```python
from build123d import *

# Parameters (mm, degrees)
SKETCH_1_R      = 24
SKETCH_1_R_2    = 3
SKETCH_1_R_3    = 2
SKETCH_1_R_4    = 1.45
SKETCH_1_R_5    = 1.5
SKETCH_1_W      = 15.1
SKETCH_1_H      = 3
SKETCH_1_W_2    = 3
SKETCH_1_H_2    = 20.1
EXTRUDE_1_DEPTH = 2
FILLET_1_R      = 10
FILLET_2_R      = 3


with BuildPart() as part:
    # 草图1 → 凸台-拉伸1 (new body)
    with BuildSketch(Plane(origin=(0, 0, 0), x_dir=(1, 0, 0), z_dir=(0, 1, 0))):
        with BuildLine():
            Line((0, -40), (-53.115531196, -40))
            Line((-53.115531196, -40), (-53.115531196, 50))
            Line((-53.115531196, 50), (23.035101229, 50))
            ThreePointArc((23.035101229, 50), (47.273662895, 61.517967257), (61.152805225, 38.549709823))
            add(Edge.make_bspline(
                [(61.152805225, 38.549709823), (43.767754296, -41.044262003), (0, -40)],
                knots=[0, 0, 0, 0.762442078, 0.762442078, 0.762442078], degree=2))
        make_face()
        with Locations(Location((0, 0, 0), (0, 0, 270))):
            Circle(SKETCH_1_R, mode=Mode.SUBTRACT)
        with Locations(Location((41.5198, 42.363514464, 0), (0, 0, 270))):
            Circle(SKETCH_1_R_2, mode=Mode.SUBTRACT)
        with Locations(Location((46, 9, 0), (0, 0, 270))):
            Circle(SKETCH_1_R_3, mode=Mode.SUBTRACT)
        with Locations(Location((-45, 40, 0), (0, 0, 270))):
            Circle(SKETCH_1_R_3, mode=Mode.SUBTRACT)
        with Locations(Location((-45, -35, 0), (0, 0, 270))):
            Circle(SKETCH_1_R_3, mode=Mode.SUBTRACT)
        with Locations(Location((35.862945751, 48.020368713, 0), (0, 0, 270))):
            Circle(SKETCH_1_R_4, mode=Mode.SUBTRACT)
        with Locations(Location((47.176654249, 48.020368713, 0), (0, 0, 270))):
            Circle(SKETCH_1_R_4, mode=Mode.SUBTRACT)
        with Locations(Location((47.176654249, 36.706660215, 0), (0, 0, 270))):
            Circle(SKETCH_1_R_4, mode=Mode.SUBTRACT)
        with Locations(Location((35.862945751, 36.706660215, 0), (0, 0, 270))):
            Circle(SKETCH_1_R_4, mode=Mode.SUBTRACT)
        with Locations(Location((-45, 22, 0), (0, 0, 270))):
            Circle(SKETCH_1_R_5, mode=Mode.SUBTRACT)
        with Locations(Location((-45, -22, 0), (0, 0, 270))):
            Circle(SKETCH_1_R_5, mode=Mode.SUBTRACT)
        with Locations(Location((34.183542703, 14.159286998, 0), (0, 0, 270))):
            Circle(SKETCH_1_R_5, mode=Mode.SUBTRACT)
        with Locations(Location((34.183542703, -14.159286998, 0), (0, 0, 270))):
            Circle(SKETCH_1_R_5, mode=Mode.SUBTRACT)
        with Locations(Location((14.159286998, -34.183542703, 0), (0, 0, 270))):
            Circle(SKETCH_1_R_5, mode=Mode.SUBTRACT)
        with Locations(Location((-14.159286998, -34.183542703, 0), (0, 0, 270))):
            Circle(SKETCH_1_R_5, mode=Mode.SUBTRACT)
        with Locations(Location((-34.183542703, -14.159286998, 0), (0, 0, 270))):
            Circle(SKETCH_1_R_5, mode=Mode.SUBTRACT)
        with Locations(Location((-34.183542703, 14.159286998, 0), (0, 0, 270))):
            Circle(SKETCH_1_R_5, mode=Mode.SUBTRACT)
        with Locations(Location((-14.159286998, 34.183542703, 0), (0, 0, 270))):
            Circle(SKETCH_1_R_5, mode=Mode.SUBTRACT)
        with Locations(Location((14.159286998, 34.183542703, 0), (0, 0, 270))):
            Circle(SKETCH_1_R_5, mode=Mode.SUBTRACT)
        with Locations(Location((-10, 47, 0), (0, 0, 270))):
            Circle(SKETCH_1_R_5, mode=Mode.SUBTRACT)
        with Locations((-31.49510891, 44.033375725)):
            Rectangle(SKETCH_1_W, SKETCH_1_H, mode=Mode.SUBTRACT)
        with Locations((13.50489109, 44)):
            Rectangle(SKETCH_1_W, SKETCH_1_H, mode=Mode.SUBTRACT)
        with Locations((-45, 0.135026031)):
            Rectangle(SKETCH_1_W_2, SKETCH_1_H_2, mode=Mode.SUBTRACT)
        Polygon((-38, 38), (-38, 18), (-23, 38), align=None, mode=Mode.SUBTRACT)
        Polygon((-38, -38), (-38, -18), (-23, -38), align=None, mode=Mode.SUBTRACT)
    extrude(amount=EXTRUDE_1_DEPTH)

    # 圆角1
    fillet_1_edges = [part.edges().sort_by_distance(p)[0] for p in [
        (-53.115531196, 1, -50),
    ]]
    fillet(fillet_1_edges, radius=FILLET_1_R)

    # 圆角2
    fillet_2_edges = [part.edges().sort_by_distance(p)[0] for p in [
        (-23, 1, -38),
        (-38, 1, -38),
        (-38, 1, -18),
        (-38, 1, 38),
        (-23, 1, 38),
        (-38, 1, 18),
    ]]
    fillet(fillet_2_edges, radius=FILLET_2_R)


solid = part.part
```
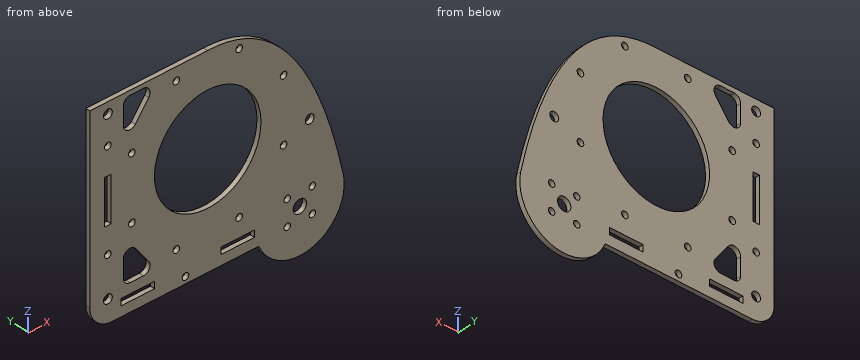
Geometry: final body of the model. Coordinates: model frame, mm. Round coordinates to 2 decimals unless told otherwise and drop trailing zeros. Answer in a Markdown table with one row per item. Add a question column.
(1) Ray query, L1, parallel to Z at x = 9.5, y = 0.6; L2, parallel to X at y = 1, z = 7.5; L3, parallel to X at y = 1.8, z = 15.5. Return the intervals inside material, ascending.
(2) Contact query for flat-ended pins moving along their axis: pin 1 (4 mm diameter, centred on x = 47.18, z = -48.02, fed in from +Y); pin 2 (1 mm diameter, centred on x = 23.5, y = 0.5, fed in from -Z); pin 3 (0.6 mm diameter, centred on x = -32.5, y = 1.5, fed in from +Z); pin 4 (2.5 mm diameter, centred on x = -45, z = 22, fed in from -Y). Output: stop coordinate, or through.
(3) Cut plane A-A, the plane z = 22. Give the number of separate pieces and of enclosed holes in the cut face, then the cut area to 3 significant figures.
Established:
| question | item | result |
|---|---|---|
| 1 | L1 | -50 to -45.5, -42.5 to -22.04, 22.04 to 39.22 |
| 1 | L2 | -53.12 to -46.5, -43.5 to -22.8, 22.8 to 45.64 |
| 1 | L3 | -53.12 to -34.86, -33.51 to -18.32, 18.32 to 33.51, 34.86 to 41 |
| 2 | pin 1 | y = 2 |
| 2 | pin 2 | z = -52.01 |
| 2 | pin 3 | z = 40 |
| 2 | pin 4 | through |
| 3 | separate pieces | 3 |
| 3 | enclosed holes | 0 |
| 3 | area | 134 mm² |
